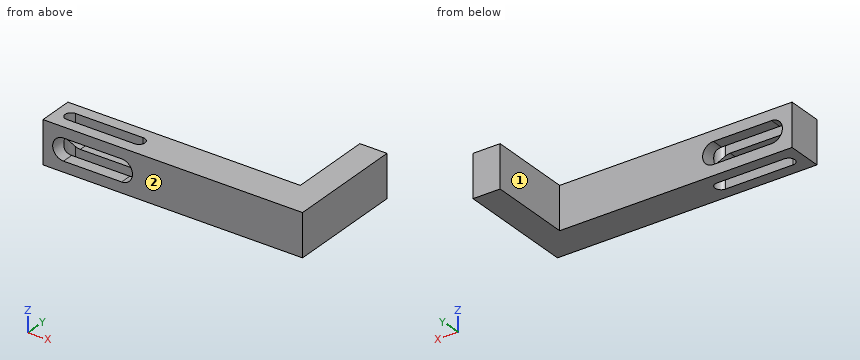
```python
from build123d import *

# Parameters (mm, degrees)
BOSS_EXTRUDE1_DEPTH = 11
CUT_EXTRUDE1_DEPTH  = 75.432855649
CUT_EXTRUDE2_DEPTH  = 75.432855649


with BuildPart() as part:
    # Sketch1 → Boss-Extrude1 (new body)
    with BuildSketch(Plane.XY):
        Polygon((0, 0), (67, 0), (67, 30.5), (60, 30.5), (60, 9), (0, 9), align=None)
    extrude(amount=-BOSS_EXTRUDE1_DEPTH)

    # Sketch2 → Cut-Extrude1 (cut, through all)
    with BuildSketch(Plane.XZ):
        with BuildLine():
            Line((5.3, -2.7), (20.3, -2.7))
            ThreePointArc((20.3, -2.7), (23.1, -5.5), (20.3, -8.3))
            Line((20.3, -8.3), (5.3, -8.3))
            ThreePointArc((5.3, -8.3), (2.5, -5.5), (5.3, -2.7))
        make_face()
    extrude(amount=-CUT_EXTRUDE1_DEPTH, mode=Mode.SUBTRACT)

    # Sketch3 → Cut-Extrude2 (cut, through all)
    with BuildSketch(Plane.XY):
        with BuildLine():
            Line((4.05, 6.05), (21.55, 6.05))
            ThreePointArc((21.55, 6.05), (23.1, 4.5), (21.55, 2.95))
            Line((21.55, 2.95), (4.05, 2.95))
            ThreePointArc((4.05, 2.95), (2.5, 4.5), (4.05, 6.05))
        make_face()
    extrude(amount=-CUT_EXTRUDE2_DEPTH, mode=Mode.SUBTRACT)


solid = part.part
```
The listing builds one solid part. Answer for the finished solid, in the listing's coordinates (mm). Face numbers are marked on the shaded views. A direction names the side the tool comes from. Round coordinates to 2 decimals unless told otherwise and drop trailing zeros. Write each loop counter-clockwise with the first axis right and the second up, starting at its lowest first coordinate (ties: lowest second). Pieces come first, ordered by that corner, then holes. Notation, with made-up numbers: (-39, -19) -> (-10, -19) arc R15 ccw to (-10, 9) -> close; hole circle Ø9 at (6.5, -31). An arc over 180 degrees is marked (long way). Answer as a JSON object with one key per item and string values. Group by question number.
Q1. Section D-D (y = 10) is taken. Write down the section's boundary in (x, z).
Q2. Straight lines are drawn through the part: line 1 along Y through (x, z) = (17, -2); line 2 along Y through (x, z) = (25.5, -0.5); line 3 along X through (y, z) = (29.5, -8.25). For each, find the intervals that lie inside material, in ascending order.
Q3. Section C-C (z = -6.25) is taken. Write down the section's boundary in (x, y), plus the area to 3 significant figures.
Q4. Each of these flat-tipped pins is pushed along its axis until it touches: pin 1 Ø3.5 at (x, z) = (12, -2) entering from +Y; pin 2 Ø2 at (y, z) = (20, -9.5) entering from -X. Where does it stop, or does it pass through?
Q5. Section B-B (x = 19.5) is taken. Write down the section's boundary in (y, z), plus the area to 3 significant figures.
Q6. Section A-A (z = -1.25) is taken. Write down the section's boundary in (x, y).
Q7. Which of the six approach directions +Z, -Z, +X, -X, +Y, -Y give full straight-line access (tool end or side, diameter ignored) to the marked faces 1 and 2?
Check values:
{
 "1": {"outline": "(60, -11) -> (67, -11) -> (67, 0) -> (60, 0) -> close"},
 "2": {"line 1": "0 to 2.95, 6.05 to 9", "line 2": "0 to 9", "line 3": "60 to 67"},
 "3": {"outline": "(0, 0) -> (2.6, 0) -> (2.6, 3.95) arc R1.55 cw to (2.6, 5.05) -> (2.6, 9) -> (0, 9) -> close; (23, 0) -> (67, 0) -> (67, 30.5) -> (60, 30.5) -> (60, 9) -> (23, 9) -> (23, 5.05) arc R1.55 cw to (23, 3.95) -> close", "area": "570 mm^2"},
 "4": {"pin 1": "y = 9", "pin 2": "x = 60"},
 "5": {"outline": "(0, -11) -> (2.95, -11) -> (2.95, -8.3) -> (0, -8.3) -> close; (0, -2.7) -> (2.95, -2.7) -> (2.95, 0) -> (0, 0) -> close; (6.05, -11) -> (9, -11) -> (9, -8.3) -> (6.05, -8.3) -> close; (6.05, -2.7) -> (9, -2.7) -> (9, 0) -> (6.05, 0) -> close", "area": "31.9 mm^2"},
 "6": {"outline": "(0, 0) -> (67, 0) -> (67, 30.5) -> (60, 30.5) -> (60, 9) -> (0, 9) -> close; hole (4.05, 2.95) -> (21.55, 2.95) arc R1.55 ccw to (21.55, 6.05) -> (4.05, 6.05) arc R1.55 ccw to start"},
 "7": {"face 1": "+Z, -Z, -X, +Y", "face 2": "+Z, -Z, +X, -X, -Y"}
}
